For this review, take the finished solid that the model builds, in its own axes (mm). Face numbers are marked on the shaded views. Round coordinates to 2 decimals unless told otherwise and drop trailing zeros. Order: outer loops, then holes, each group sorted by start corner. A loop starts at its lowest first (then second) coordinate and runs counter-clockwise, first axis right, second up. Notation, with made-up numbers: (-7.75, 65.5) -> (5.25, 65.5) arc R17 ccw to (5.25, 72.5) -> close; hole circle Ø3 at (78, -2.75). An arc over 180 degrees is marked (long way). Use a Markdown table: item, result. Add a question column.
1) Consider section D-D (y = 16.75). State the section outline as (x, z) points, plus the area to 3 significant figures.
2) Draft analysis for pull direction X (two halves, no side actions). For the marked faces 1, 2 and 3, state which applies: pulls with the +X half, pulls with the -X half, needs draft (parallel to the pull), parting line crosses it, or undercut.
3) Consider section C-C (x = 36.5). State the section outline as (y, z) points, plus the area to 3 significant figures.
4) Clearance check with flat-ended pins moving along their axes: P1, Ø5.5, axis at x = 64.25, y = 16.75, coming from the -Z side; P2, Ø2, axis at x = 65, y = 5, coming from the +Z side; P3, Ø4, axis at x = 65, y = 55, coming from the +Z side. State where each tip first meets the part, or that it passes through.
5) Consider section A-A (y = 32.5). State the section outline as (x, z) points.
6) Consider section B-B (z = 1.9). Give the number of separate pieces and of enclosed holes in the cut face, plus the area to 3 significant figures.
7) Wall thickness on line 1 along X through (y, z) = (16.75, 4.15); line 2 along Y through (x, z) = (24.5, 0.45); line 3 along X through (y, z) = (48.5, 4.2): over which ranges is each line inside the solid? List them lowest first. Write a range as [from, to].
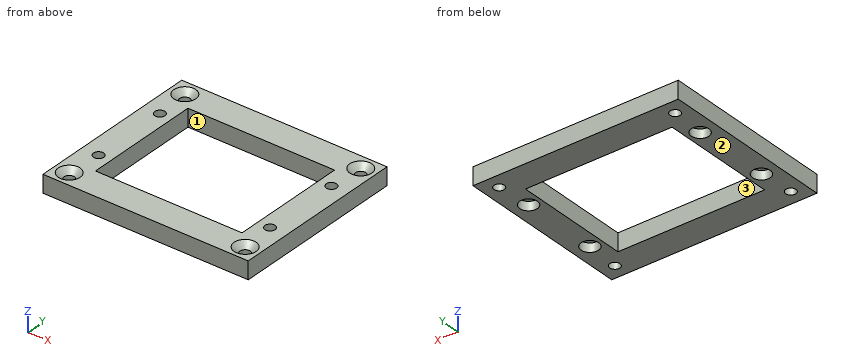
```python
from build123d import *

# Parameters (mm, degrees)
SKETCH1_W           = 70
SKETCH1_H           = 60
SKETCH1_R           = 1.75
SKETCH1_W_2         = 50
SKETCH1_H_2         = 40
BOSS_EXTRUDE1_DEPTH = 6
CHAMFER1_SIZE       = 2
SKETCH3_R           = 3
CUT_EXTRUDE1_DEPTH  = 3


with BuildPart() as part:
    # Sketch1 → Boss-Extrude1 (new body)
    with BuildSketch(Plane.XY):
        with Locations((35, 30)):
            Rectangle(SKETCH1_W, SKETCH1_H)
        with Locations((5.75, 16.75)):
            Circle(SKETCH1_R, mode=Mode.SUBTRACT)
        with Locations((5.75, 43.25)):
            Circle(SKETCH1_R, mode=Mode.SUBTRACT)
        with Locations((64.25, 43.25)):
            Circle(SKETCH1_R, mode=Mode.SUBTRACT)
        with Locations((64.25, 16.75)):
            Circle(SKETCH1_R, mode=Mode.SUBTRACT)
        with Locations((5, 55)):
            Circle(SKETCH1_R, mode=Mode.SUBTRACT)
        with Locations((65, 55)):
            Circle(SKETCH1_R, mode=Mode.SUBTRACT)
        with Locations((65, 5)):
            Circle(SKETCH1_R, mode=Mode.SUBTRACT)
        with Locations((5, 5)):
            Circle(SKETCH1_R, mode=Mode.SUBTRACT)
        with Locations((35, 30)):
            Rectangle(SKETCH1_W_2, SKETCH1_H_2, mode=Mode.SUBTRACT)
    extrude(amount=BOSS_EXTRUDE1_DEPTH)

    # Chamfer1
    chamfer1_edges = [part.edges().sort_by_distance(p)[0] for p in [
        (3.25, 55, 6),
        (63.25, 55, 6),
        (63.25, 5, 6),
        (3.25, 5, 6),
    ]]
    chamfer(chamfer1_edges, length=CHAMFER1_SIZE)

    # Sketch3 → Cut-Extrude1 (cut)
    with BuildSketch(Plane(origin=(0, 0, 0), x_dir=(-1, 0, 0), z_dir=(0, 0, -1))):
        with Locations((-64.25, 43.25)):
            Circle(SKETCH3_R)
        with Locations((-64.25, 16.75)):
            Circle(SKETCH3_R)
        with Locations((-5.75, 16.75)):
            Circle(SKETCH3_R)
        with Locations((-5.75, 43.25)):
            Circle(SKETCH3_R)
    extrude(amount=-CUT_EXTRUDE1_DEPTH, mode=Mode.SUBTRACT)


solid = part.part
```
Results list:
| question | item | result |
|---|---|---|
| 1 | outline | (0, 0) -> (2.75, 0) -> (2.75, 3) -> (4, 3) -> (4, 6) -> (0, 6) -> close; (7.5, 3) -> (8.75, 3) -> (8.75, 0) -> (10, 0) -> (10, 6) -> (7.5, 6) -> close; (60, 0) -> (61.25, 0) -> (61.25, 3) -> (62.5, 3) -> (62.5, 6) -> (60, 6) -> close; (66, 3) -> (67.25, 3) -> (67.25, 0) -> (70, 0) -> (70, 6) -> (66, 6) -> close |
| 1 | area | 63.0 mm2 |
| 2 | face 1 | undercut |
| 2 | face 2 | needs draft |
| 2 | face 3 | undercut |
| 3 | outline | (0, 0) -> (10, 0) -> (10, 6) -> (0, 6) -> close; (50, 0) -> (60, 0) -> (60, 6) -> (50, 6) -> close |
| 3 | area | 120 mm2 |
| 4 | P1 | z = 3 |
| 4 | P2 | through |
| 4 | P3 | z = 4.25 |
| 5 | outline | (0, 0) -> (10, 0) -> (10, 6) -> (0, 6) -> close; (60, 0) -> (70, 0) -> (70, 6) -> (60, 6) -> close |
| 6 | separate pieces | 1 |
| 6 | enclosed holes | 9 |
| 6 | area | 2,050 mm2 |
| 7 | line 1 | [0, 4], [7.5, 10], [60, 62.5], [66, 70] |
| 7 | line 2 | [0, 10], [50, 60] |
| 7 | line 3 | [0, 10], [60, 70] |
